For this review, take the finished solid that the model builds, in its own axes (mm). Face numbers are marked on the shaded views. A direction names the side the tool comes from. Give positions to 0.01 mm unless a question says otherwise; leave off trailing zeros. Write each loop counter-clockwise with the first axis right and the second up, starting at its lowest first coordinate (ties: lowest second). Pieces come first, ordered by that corner, then holes.
Q1. For line 1 (Y direction, x = 0, z = 6.35); line 2 (Y direction, x = -7.5, z = 6.5); line 3 (X direction, y = -6.5, z = 5), list the stretches that pass through material, from the lowest coordinate up.
Q2. Mouldability with a two-part tool opening along Y and no side actions: class the marked faces 3, 4, 5 and 6 as released by +Y, released by -Y, zero draft, split by the parting line, or undercut.
Q3. We need section D-D (x = -12). Write out the cut boundary in (y, z).
Q4. Machinability: for the marked faces 1 and 2, which of the approach directions +Z, -Z, +X, -X, +Y, -Y give a long, thin tool a straight path to every point of the face, cutting with its end or side? Answer none if there is none.
Q5. Insertion check: P1, Ø2, axis at x = 4, y = 12.5, coming from the -Z side; P2, Ø2, axis at y = 7, z = 4, coming from the -X side; P3, Ø4, axis at x = 12, z = 3, coming from the -Y side; P4, Ø1.5, axis at x = -3.5, z = 1, coming from the +Y side. Each pin has a flat end and moves straight along its axis. Give the tip position at first contact, or say it passes through.
Q6. We need section C-C (z = 4.5). Write out the cut boundary in (x, y), then the cut area to 3 significant figures.
Q7. We need section A-A (y = 0). Write out the cut boundary in (x, z), then the cut area to 3 significant figures.
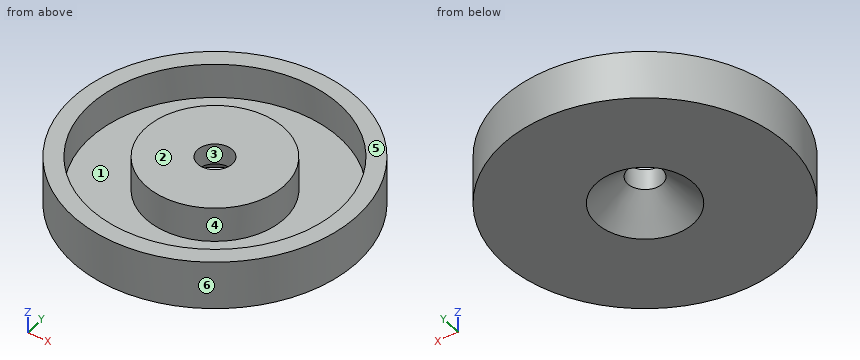
```python
from build123d import *

# Parameters (mm, degrees)
F0_R     = 20.5
F1_DEPTH = 7
F2_R     = 18
F2_R_2   = 10
F3_DEPTH = 5
F4_R     = 2.5
F5_DEPTH = 7.001
F6_SIZE2 = 4
F6_SIZE  = 4.5


with BuildPart() as f1:
    # F0 (on Top) → F1 (new body)
    with BuildSketch(Plane.XY):
        Circle(F0_R)
    extrude(amount=F1_DEPTH)

    # F2 (on face) → F3 (cut)
    with BuildSketch(Plane.XY.offset(7)):
        Circle(F2_R)
        Circle(F2_R_2, mode=Mode.SUBTRACT)
    extrude(amount=-F3_DEPTH, mode=Mode.SUBTRACT)

    # F4 (on face) → F5 (cut, through all)
    with BuildSketch(Plane.XY.offset(7)):
        Circle(F4_R)
    extrude(amount=-F5_DEPTH, mode=Mode.SUBTRACT)

    # F6
    f6_edges = [f1.edges().sort_by_distance(p)[0] for p in [
        (-2.5, 0, 0),
    ]]
    chamfer(f6_edges, length=F6_SIZE, length2=F6_SIZE2)


solid = f1.part
```
Computed:
1. line 1: y = -20.5 to -18, -10 to -2.5, 2.5 to 10, 18 to 20.5
1. line 2: y = -19.08 to -16.36, -6.61 to 6.61, 16.36 to 19.08
1. line 3: x = -19.44 to -16.79, -7.6 to 7.6, 16.79 to 19.44
2. face 3: undercut
2. face 4: undercut
2. face 5: zero draft
2. face 6: split by the parting line
3. outline: (-16.62, 0) - (16.62, 0) - (16.62, 7) - (13.42, 7) - (13.42, 2) - (-13.42, 2) - (-13.42, 7) - (-16.62, 7) - close
4. face 1: +Z
4. face 2: +Z, +X, -X, +Y, -Y
5. P1: stops at z = 0
5. P2: stops at x = -19.6
5. P3: stops at y = -17.9
5. P4: stops at y = 20.31
6. outline: circle Ø41 at (0, 0); circle Ø20 at (0, 0); hole circle Ø36 at (0, 0); hole circle Ø5 at (0, 0)
6. area: 597 mm2
7. outline: (-20.5, 0) - (-7, 0) - (-2.5, 4) - (-2.5, 7) - (-10, 7) - (-10, 2) - (-18, 2) - (-18, 7) - (-20.5, 7) - close; (2.5, 4) - (7, 0) - (20.5, 0) - (20.5, 7) - (18, 7) - (18, 2) - (10, 2) - (10, 7) - (2.5, 7) - close
7. area: 154 mm2
